from build123d import *

# Parameters (mm, degrees)
F0_W     = 45
F0_H     = 45
F1_DEPTH = 10
F2_W     = 6
F2_H     = 27
F3_DEPTH = 4510
F4_R     = 4.5
F4_R_2   = 1.5
F5_DEPTH = 10
F6_W     = 27
F6_H     = 38.457482
F7_DEPTH = 5


with BuildPart() as f1:
    # F0 (on Right) → F1 (new body)
    with BuildSketch(Plane.YZ):
        with Locations((22.498396, 22.80707)):
            Rectangle(F0_W, F0_H)
    extrude(amount=F1_DEPTH)

    # F2 (on Top) → F3 (cut)
    with BuildSketch(Plane.XY):
        with Locations((5, 22.498396)):
            Rectangle(F2_W, F2_H)
    extrude(amount=F3_DEPTH, mode=Mode.SUBTRACT)

    # F4 (on Right) → F5 (cut)
    with BuildSketch(Plane.YZ):
        with Locations((22.498396, 20.30707)):
            Circle(F4_R)
        with Locations((4.998396, 28.30707)):
            Circle(F4_R_2)
        with Locations((39.998396, 28.30707)):
            Circle(F4_R_2)
    extrude(amount=F5_DEPTH, mode=Mode.SUBTRACT)

    # F6 (on face) → F7 (cut)
    with BuildSketch(Plane.YZ.offset(10)):
        with Locations((22.498396, 22.910485)):
            Rectangle(F6_W, F6_H)
    extrude(amount=-F7_DEPTH, mode=Mode.SUBTRACT)


solid = f1.part
Input: part model. Units: mm. Frame: model coordinates. A direction names the side the tool comes from. Give positions to 0.01 mm unless a question says otherwise; leave off trailing zeros. Loops run counter-clockwise (first coordinate to the right, second up) from the corner with the lowest first, then second, coordinate; pieces in that order, holes last. Notation, with made-up numbers: (24.25, 62.5) - (73.25, 62.5) arc R30 cw to (73.25, 96.5) - close; hole circle Ø10 at (36.5, -8). An arc over 180 degrees is marked (long way). Use CSV: the item, a comma, the result in double quotes. Start each with the question number.
Item 1: Section A-A on y = 15.5. Return loops of the section in (x, z), then the cut area to 3 significant figures.
Item 2: Contact query for flat-ended pins moving along their axis: P1, Ø1, axis at y = 20.5, z = 44.5, coming from the -X side; P2, Ø2.5, axis at y = 40, z = 28.31, coming from the +X side; P3, Ø8, axis at y = 19, z = 13, coming from the +X side. Output: stop coordinate, or through.
Item 3: Section B-B on x = 2.75. Return loops of the section in (y, z), then the cut area to 3 significant figures.
Item 4: Reachability of faces 1 (the cylindrical face through (4.93, 38.81, 27.39)), 2 (the flat face through (9, 22, 42.139)), 3 (the flat face through (2, 22, 27)) from +Z, -Z, +X, -X, +Y, -Y: full face, straight path, thin tool, end or side. Return the list, or none.
Item 5: Mould query, pull axis X, two halves, no side actions, for faces 4 (the flat face through (10, 37, 23)), 5 (the flat face through (5, 44.998, 22)), 6 (the flat face through (8, 22, 44)). Classes: pulls with the +X half, pulls with the -X half, needs draft (parallel to the pull), parting line crosses it, or undercut.
Item 6: Section C-C on y = 21. Return loops of the section in (x, z).
Item 7: Section D-D on z = 18.5. Return loops of the section in (x, y), then the cut area to 3 significant figures.
Item 8: Line query: line 1 (Y direction, x = 6.75, z = 31.5); line 2 (Z direction, x = 9, y = 17); line 3 (X direction, y = 18, z = 14.5). Output: solid intervals per line, ascending.
Ans:
1,outline,"(0, 0.31) - (2, 0.31) - (2, 45.31) - (0, 45.31) - close; (8, 0.31) - (10, 0.31) - (10, 3.68) - (8, 3.68) - close; (8, 42.14) - (10, 42.14) - (10, 45.31) - (8, 45.31) - close"
1,area,"103 mm2"
2,P1,"stops at x = 0"
2,P2,"passes through"
2,P3,"stops at x = 2"
3,outline,"(0, 0.31) - (9, 0.31) - (9, 45.31) - (0, 45.31) - close; (36, 0.31) - (45, 0.31) - (45, 45.31) - (36, 45.31) - close; hole circle Ø3 at (5, 28.31); hole circle Ø3 at (40, 28.31)"
3,area,"796 mm2"
4,face 1,"+X, -X"
4,face 2,"+X"
4,face 3,"+Z, -Z"
5,face 4,"pulls with the +X half"
5,face 5,"needs draft"
5,face 6,"undercut"
6,outline,"(0, 0.31) - (2, 0.31) - (2, 16.06) - (0, 16.06) - close; (0, 24.55) - (2, 24.55) - (2, 45.31) - (0, 45.31) - close; (8, 0.31) - (10, 0.31) - (10, 3.68) - (8, 3.68) - close; (8, 42.14) - (10, 42.14) - (10, 45.31) - (8, 45.31) - close"
7,outline,"(0, 0) - (10, 0) - (10, 9) - (2, 9) - (2, 18.38) - (0, 18.38) - close; (0, 26.62) - (2, 26.62) - (2, 36) - (10, 36) - (10, 45) - (0, 45) - close"
7,area,"218 mm2"
8,line 1,"y = 0 to 9, 36 to 45"
8,line 2,"z = 0.31 to 3.68, 42.14 to 45.31"
8,line 3,"x = 0 to 2"
